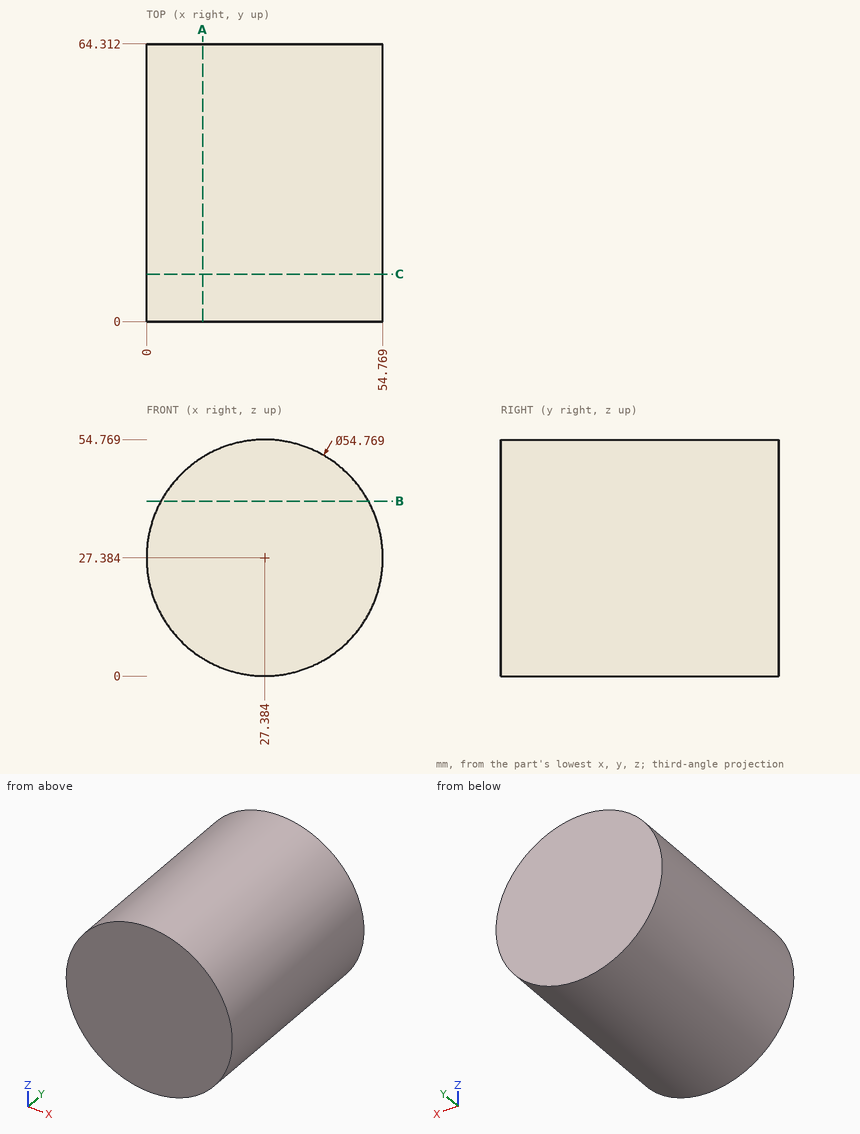
Part print with two shaded views. Sizes in mm from the minimum x, y, z corner. Round coordinates to 2 decimals unless told otherwise and drop trailing zeros. Write each loop counter-clockwise with the first axis right and the second up, starting at its lowest first coordinate (ties: lowest second). Pieces come first, ordered by that corner, then holes. Notation, with made-up numbers: M 27,-31 L 39,-31 A22 cw 39,5 Z; hole C 76.25,-29.5 d3. An arc over 180 degrees is marked long. Answer as CSV lines item,"result". Start each with the question number.
1) Band-saw the part on A-A (x = 13). List the corners of the cut face in (y, z), then the cut area to 3 significant figures.
2) Drop flat-ended pins along their axis: pin 1 (4 mm diameter, centred on y = 15, z = 44, fed in from +X); pin 2 (2 mm diameter, centred on x = 46, y = 53, fed in from +Z); pin 3 (8 mm diameter, centred on x = 32.5, y = 20, fed in from +Z). Give the stop position or say it passes through.
3) Drill centre lines: L1, parallel to Z at x = 17, y = 26 (1 decimal); L2, parallel to Z at x = 46.5, y = 59.5 (1 decimal); L3, parallel to X at y = 24, z = 12.5. Where is each one in solid material? Low to high.
4) Band-saw the part on C-C (y = 11). List the corners of the cut face in (x, z) (1 decimal).
5) Band-saw the part on B-B (z = 40.5). List the corners of the cut face in (x, y) (1 decimal), then the cut area to 3 significant figures.
Worked out:
1,outline,"M 0,4.08 L 64.31,4.08 L 64.31,50.69 L 0,50.69 Z"
1,area,"3,000 mm²"
2,pin 1,"x = 50.54"
2,pin 2,"z = 48.35"
2,pin 3,"z = 54.75"
3,L1,"2 to 52.7"
3,L2,"7.8 to 47"
3,L3,"4.4 to 50.37"
4,outline,"C 27.4,27.4 d54.8"
5,outline,"M 3.3,0 L 51.4,0 L 51.4,64.3 L 3.3,64.3 Z"
5,area,"3,090 mm²"
